The figure shows three views and two pictorial views of one solid part (mm, origin at its lowest corner). Answer the questions. Give positions to 0.01 mm unless a question says otherwise; leave off trailing zeros. Loops run counter-clockwise (first coordinate to the right, second up) from the corner with the lowest first, then second, coordinate; pieces in that order, holes last. Notation, with made-up numbers: (-39.5, 22.5) - (0.5, 22.5) arc R11 ccw to (0.5, 32.5) - close; hole circle Ø2 at (74.25, 0). An arc over 180 degrees is marked (long way). Write each question's results on one line, items separated by ' | '.
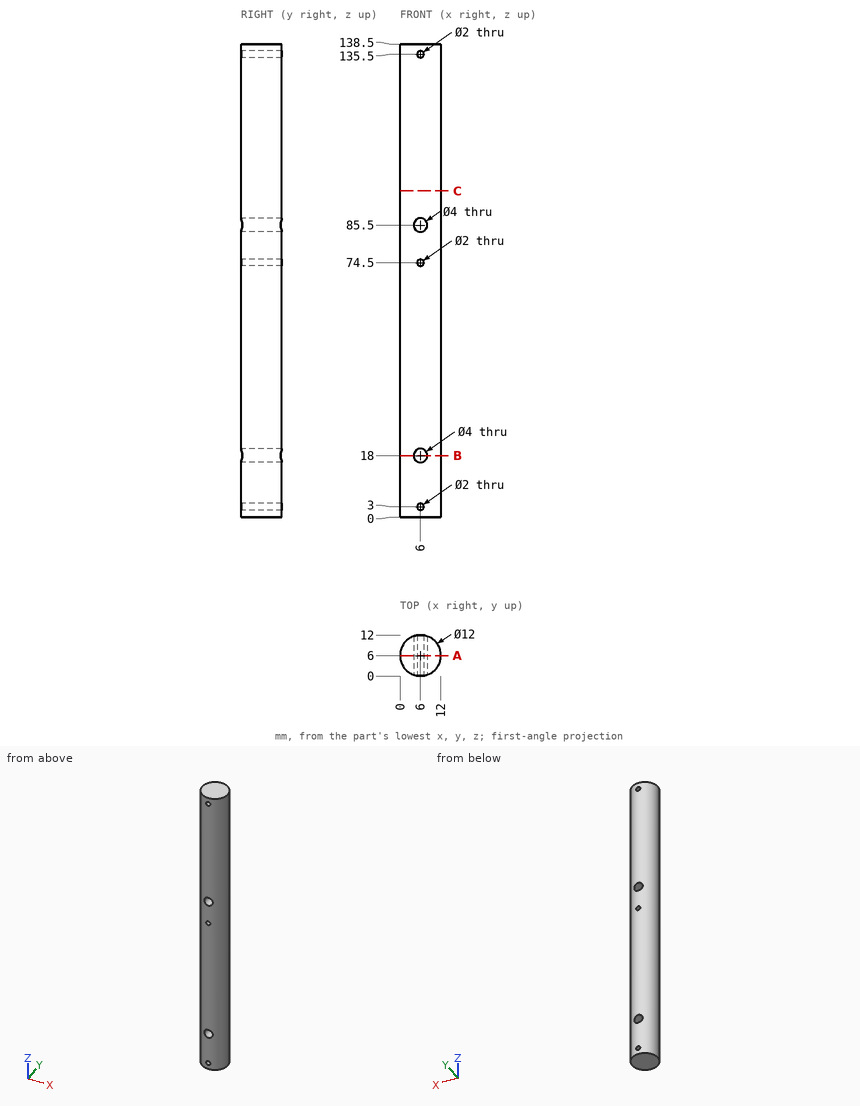
Item 1: A cutting plane is placed at B-B, the plane z = 18. Determine the outline of the cut face in (x, y), plus the area to 3 significant figures.
Values found:
outline: (4, 0.34) - (4, 11.66) arc R6 ccw to start; (8, 0.34) arc R6 ccw to (8, 11.66) - close | area: 66.0 mm²
Item 2: Flat-ended cylindrical pins translate along their axes: P1, Ø6.5, axis at x = 6, z = 85.5, coming from the -Y side; P2, Ø4, axis at y = 3.5, z = 15.5, coming from the +X side; P3, Ø2.5, axis at x = 6, z = 18, coming from the -Y side (1 decimal); P4, Ø2, axis at x = 9.5, z = 39, coming from the +Y side. Find the tip coordinate at first contact, or state that the pin passes through.
Values found:
P1: stops at y = 0 | P2: stops at x = 11.98 | P3: passes through | P4: stops at y = 11.45
Item 3: A cutting plane is placed at C-C, the plane z = 95.5. Determine the outline of the cut face in (x, y), plus the area to 3 significant figures.
Values found:
outline: circle Ø12 at (6, 6) | area: 113 mm²
Item 4: A cutting plane is placed at A-A, the plane y = 6. Determine the outline of the cut face in (x, z), plus the area to 3 significant figures.
Values found:
outline: (0, 0) - (12, 0) - (12, 138.5) - (0, 138.5) - close; hole circle Ø4 at (6, 18); hole circle Ø4 at (6, 85.5); hole circle Ø2 at (6, 3); hole circle Ø2 at (6, 74.5); hole circle Ø2 at (6, 135.5) | area: 1,630 mm²
Item 5: Find the intervals of material crossed by line 1 along Z through (x, y) = (5.75, 9.5); line 2 along Z through (x, y) = (4.5, 7); line 3 along X through (y, z) = (5.5, 85.5), in increasing order. Write a range as [from, to].
Values found:
line 1: z = [0, 2.03], [3.97, 16.02], [19.98, 73.53], [75.47, 83.52], [87.48, 134.53], [136.47, 138.5] | line 2: z = [0, 16.68], [19.32, 84.18], [86.82, 138.5] | line 3: x = [0.02, 4], [8, 11.98]
